Check sheet for the drawn part. Datum: minimum x, y, z corner. Units: mm. A direction names the side the tool comes from. Coordinates: 2 decimals unless noted, no trailing zeros. Write each loop counter-clockwise with the first axis right and the second up, starting at its lowest first coordinate (ties: lowest second). Pieces come first, ordered by that corner, then holes. Notation, with made-up numbers: (-8.75, 17) - (5.25, 17) arc R28 ccw to (5.25, 43) - close; hole circle Ø7 at (-13, -11). An arc over 180 degrees is marked (long way). Write each question's results on one line, items separated by ' | '.
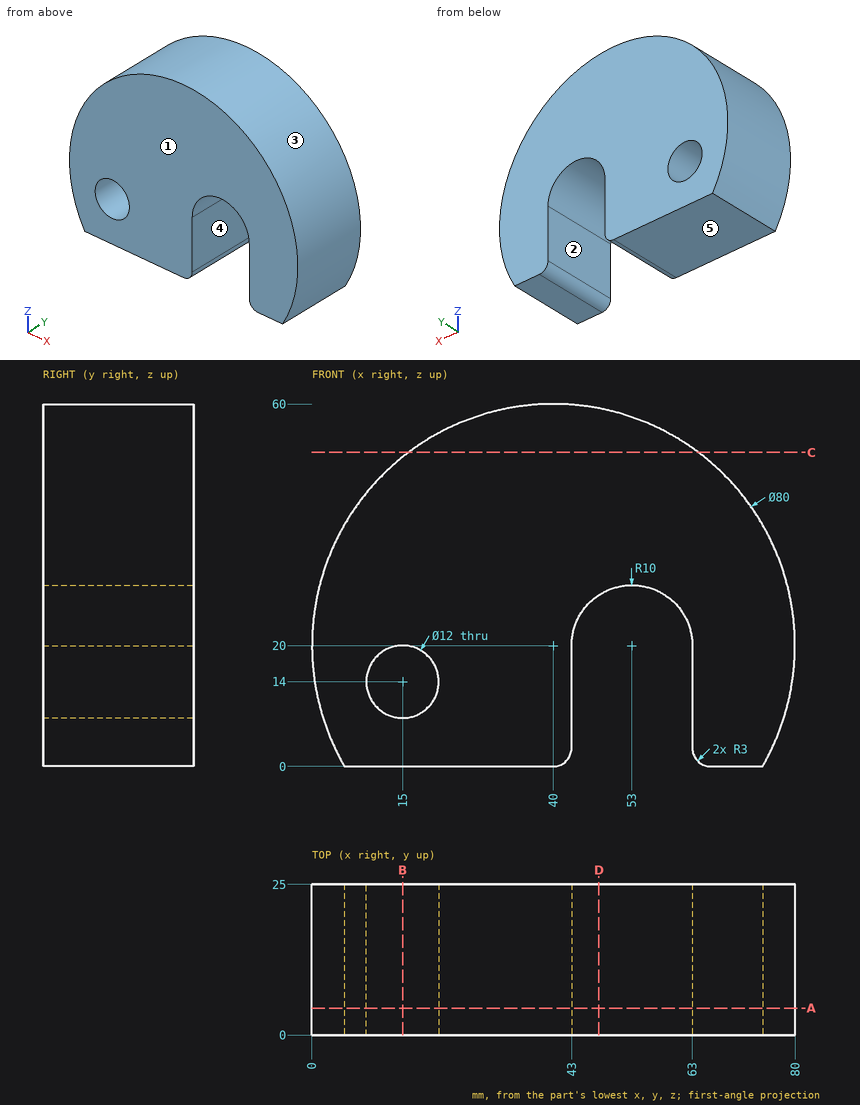
1. Sectioned sample at B-B (x = 15). Record the cut outline in (y, z) (3 decimals).
Values follow:
outline: (0, 0) - (25, 0) - (25, 8) - (0, 8) - close; (0, 20) - (25, 20) - (25, 51.225) - (0, 51.225) - close
2. Sectioned sample at C-C (z = 52). Record the cut outline in (x, y), then the cut area to 3 significant figures.
Values follow:
outline: (16, 0) - (64, 0) - (64, 25) - (16, 25) - close | area: 1,200 mm^2
3. Sectioned sample at D-D (x = 47.5). Record the cut outline in (y, z), then the cut area to 3 significant figures.
Values follow:
outline: (0, 28.35) - (25, 28.35) - (25, 59.29) - (0, 59.29) - close | area: 773 mm^2
4. Go/stop test with flat-tipped pins: pin 1 (19 mm diameter, centred on x = 15, z = 14, fed in from +Y); pin 2 (2 mm diameter, centred on x = 16.5, y = 20, fed in from +Z); pin 3 (6 mm diameter, centred on y = 10, z = 22.5, fed in from -X); pin 4 (5 mm diameter, centred on y = 18, z = 39.5, fed in from -X). Record where each tip stops, or that it passes through.
Values follow:
pin 1: stops at y = 25 | pin 2: stops at z = 53.07 | pin 3: stops at x = 0 | pin 4: stops at x = 3.79
5. Sectioned sample at A-A (y = 4.5). Record the cut outline in (x, z).
Values follow:
outline: (5.36, 0) - (40, 0) arc R3 ccw to (43, 3) - (43, 20) arc R10 cw to (63, 20) - (63, 3) arc R3 ccw to (66, 0) - (74.64, 0) arc R40 ccw (long way) to start; hole circle Ø12 at (15, 14)
6. Access from +Z, -Z, +X, -X, +Y, -Y to the whole of each face (thin tool, end or side, straight path). Record for the marked faces 1 and 2.
Values follow:
face 1: +Z, -Z, +X, -X, -Y | face 2: -Z, +Y, -Y
7. Draft check along X on the marked faces 3, 4 and 5. Enter one of: pulls with the +X half, pulls with the -X half, needs draft (parallel to the pull), parting line crosses it, or undercut.
Values follow:
face 3: parting line crosses it | face 4: undercut | face 5: needs draft
8. Material ranges on L1, parallel to X at y = 12, z = 26.5; L2, parallel to Z at x = 15, y = 13 (3 decimals); L3, parallel to Z at x = 22, y = 1.75, recorded low to high. Write a range as [from, to].
Values follow:
L1: x = [0.53, 45.4], [60.6, 79.47] | L2: z = [0, 8], [20, 51.225] | L3: z = [0, 55.72]
